Could you check a few things on this drawing? It's one solid part, dimensions in mm from its lowest x, y, z. Round coordinates to 2 decimals unless told otherwise and drop trailing zeros. Write each loop counter-clockwise with the first axis right and the second up, starting at its lowest first coordinate (ties: lowest second). Pieces come first, ordered by that corner, then holes. Notation, with made-up numbers: (19, 52.25) - (64, 52.25) arc R34 cw to (64, 89.25) - close; hole circle Ø5 at (79, -13.5). An arc over 180 degrees is marked (long way). Use one line per item in the form item = value. Start each with the question number.
1. I want a section at C-C, the plane x = 6.35. List the corners of the cut face in (y, z) for me, plus the area to 3 significant figures.
2. We'd pull the mould along X, two halves only. Please class the marked faces 1, 2 and 3: +X half, -X half, draft (parallel to the pull), parting line (faces both ways), or undercut.
3. I want a section at A-A, the plane z = 6.35. State how many separate pieces and enclosed holes the cut face has, plus the area to 3 significant figures.
4. If I drill on line 1 along X through (y, z) = (5.5, 6.35); line 2 along X through (y, z) = (9.5, 6.25); line 3 along X through (y, z) = (5.25, 2), over which ranges is the centre line in solid material (lowest first)?
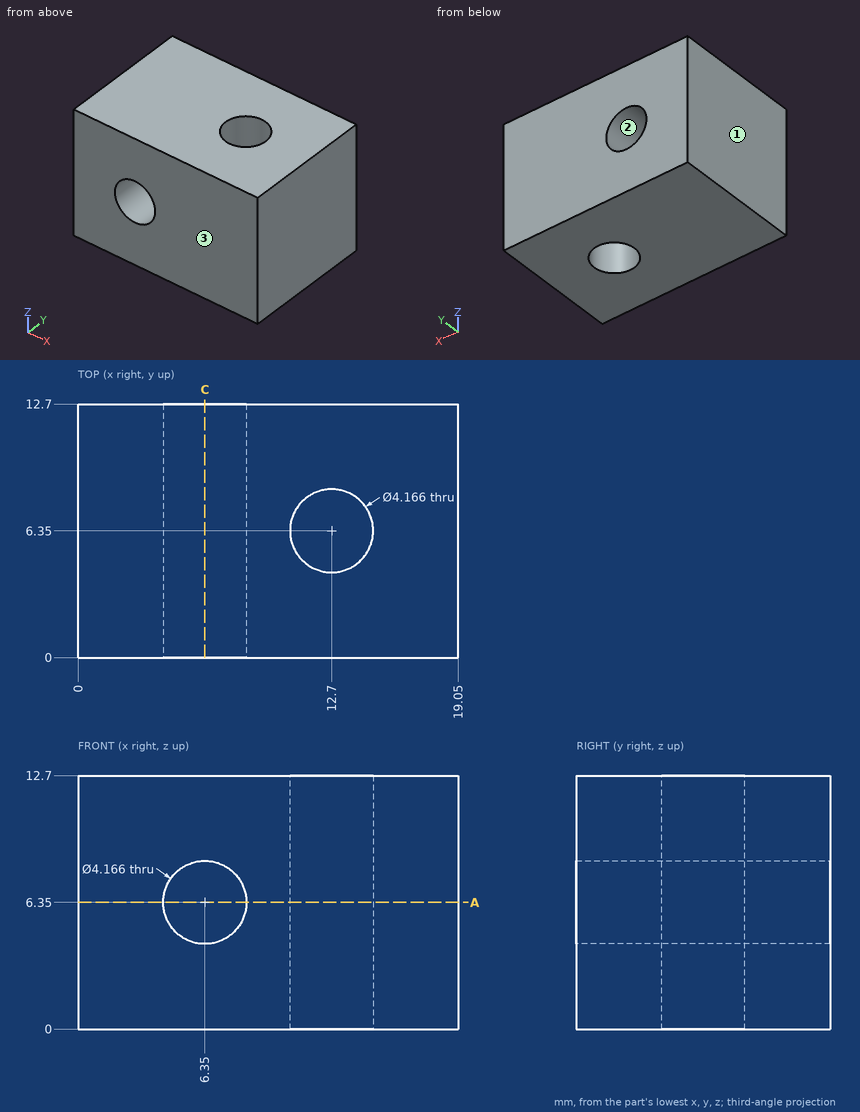
Model answer:
q1.outline = (0, 0) - (12.7, 0) - (12.7, 4.27) - (0, 4.27) - close; (0, 8.43) - (12.7, 8.43) - (12.7, 12.7) - (0, 12.7) - close
q1.area = 108 mm2
q2.face_1 = -X half
q2.face_2 = undercut
q2.face_3 = draft
q3.separate_pieces = 2
q3.enclosed_holes = 1
q3.area = 175 mm2
q4.line_1 = 0 to 4.27, 8.43 to 10.8, 14.6 to 19.05
q4.line_2 = 0 to 4.27, 8.43 to 19.05
q4.line_3 = 0 to 10.93, 14.47 to 19.05
